```python
from build123d import *

# Parameters (mm, degrees)
SKETCH1_R           = 2.15
BOSS_EXTRUDE1_DEPTH = 4
FILLET1_R           = 2
FILLET3_R           = 1


with BuildPart() as part:
    # Sketch1 → Boss-Extrude1 (new body)
    with BuildSketch(Plane.XY):
        with BuildLine():
            Line((-5e-09, -4), (50.8, -4))
            ThreePointArc((50.8, -4), (53.628427143, -2.828427107), (54.8, 5.1e-08))
            Line((54.8, 5.1e-08), (54.8, 38.1))
            ThreePointArc((54.8, 38.1), (52.588854382, 41.677708764), (48.4, 41.3))
            Line((48.4, 41.3), (25.4, 24.05))
            Line((25.4, 24.05), (2.4, 41.3))
            ThreePointArc((2.4, 41.3), (-1.788854382, 41.677708764), (-4, 38.1))
            Line((-4, 38.1), (-4, 0))
            ThreePointArc((-4, 0), (-2.828427127, -2.828427123), (-5e-09, -4))
        make_face()
        Polygon((46.8, 8), (32.066666667, 19.05), (46.8, 30.1), align=None, mode=Mode.SUBTRACT)
        Circle(SKETCH1_R, mode=Mode.SUBTRACT)
        Polygon((4, 8), (4, 30.1), (18.733333333, 19.05), align=None, mode=Mode.SUBTRACT)
        Polygon((25.4, 14.05), (38.8, 4), (12, 4), align=None, mode=Mode.SUBTRACT)
        with Locations((25.4, 19.05)):
            Circle(SKETCH1_R, mode=Mode.SUBTRACT)
        with Locations((50.8, 0)):
            Circle(SKETCH1_R, mode=Mode.SUBTRACT)
        with Locations((0, 38.1)):
            Circle(SKETCH1_R, mode=Mode.SUBTRACT)
        with Locations((50.8, 38.1)):
            Circle(SKETCH1_R, mode=Mode.SUBTRACT)
    extrude(amount=BOSS_EXTRUDE1_DEPTH)

    # Fillet1
    fillet1_edges = [part.edges().sort_by_distance(p)[0] for p in [
        (18.733333333, 19.05, 2),
        (25.4, 14.05, 2),
        (32.066666667, 19.05, 2),
        (25.4, 24.05, 2),
    ]]
    fillet(fillet1_edges, radius=FILLET1_R)

    # Fillet3
    fillet3_edges = [part.edges().sort_by_distance(p)[0] for p in [
        (4, 30.1, 2),
        (4, 8, 2),
        (12, 4, 2),
        (38.8, 4, 2),
        (46.8, 30.1, 2),
        (46.8, 8, 2),
    ]]
    fillet(fillet3_edges, radius=FILLET3_R)


solid = part.part
```
Geometry: final body of the model. Coordinates: model frame, mm. A direction names the side the tool comes from. Give positions to 0.01 mm unless a question says otherwise; leave off trailing zeros. Order: outer loops, then holes, each group sorted by start corner. A loop starts at its lowest first (then second) coordinate and runs counter-clockwise, first axis right, second up. Notation, with made-up numbers: (75, 64) -> (91, 64) arc R26 cw to (91, 84) -> close; hole circle Ø1 at (18, 46). An arc over 180 degrees is marked (long way). Write each question's results on one line, items separated by ' | '. Start each with the question number.
1) Section C-C (z = 0.7). Count the separate pieces of the cut face and the enclosed holes in it, then the cut area to 3 significant figures.
2) Section D-D (x = 25.4). Return loops of the section in (y, z).
3) First-contact query: pin 1 (1.5 mm diameter, centred on x = 11, y = 30.5, fed in from -Z); pin 2 (2 mm diameter, centred on x = 20.5, z = 1.5, fed in from +Y) (3 decimals); pin 3 (1 mm diameter, centred on x = 21, z = 3, fed in from +Y) (3 decimals); pin 4 (1 mm diameter, centred on x = 36, z = 1, fed in from +Y) (3 decimals). Flat tips, straight axial feed; report the tip coordinate or a pass-through.
4) Line query: line 1 (Y direction, x = 0, z = 1); line 2 (Y direction, x = 25.4, z = 1); line 3 (X direction, y = 27, z = 0.8). Output: solid intervals per line, ascending. Write a range as from..to.
5) Draft query along X for faces 1 (the flat face through (25, -4, 2)), 2 (the flat face through (54.8, 19, 2)), 3 (the cylindrical face through (46.26, 9.11, 2.03)). Return one class per face: pulls with the +X half, pulls with the -X half, needs draft (parallel to the pull), parting line crosses it, or undercut.
6) Section B-B (y = 12). Return loops of the section in (x, z), then the cut area to 3 significant figures.
7) Section A-A (x = 13). Return loops of the section in (y, z).
8) Set-up query: faces 4 (the flat face through (37.653, 33.239, 1.972)), 5 (the cylindrical face through (14, 5, 2)), 6 (the cylindrical face through (-2.859, -2.797, 1.972)). Return all of +Z, -Z, +X, -X, +Y, -Y with unobstructed straight access to the full face (end or side cutting, diameter ignored); none if empty.
Calculated:
1) separate pieces: 1 | enclosed holes: 8 | area: 1,740 mm2
2) outline: (-4, 0) -> (4, 0) -> (4, 4) -> (-4, 4) -> close; (13.55, 0) -> (16.9, 0) -> (16.9, 4) -> (13.55, 4) -> close; (21.2, 0) -> (24.55, 0) -> (24.55, 4) -> (21.2, 4) -> close
3) pin 1: z = 0 | pin 2: y = 28.475 | pin 3: y = 27.725 | pin 4: y = 32.375
4) line 1: -4..-2.15, 2.15..35.95, 40.25..42.1 | line 2: -4..4, 13.55..16.9, 21.2..24.55 | line 3: -4..4, 8.13..21.47, 29.33..42.67, 46.8..54.8
5) face 1: needs draft | face 2: pulls with the +X half | face 3: undercut
6) outline: (-4, 0) -> (4, 0) -> (4, 4) -> (-4, 4) -> close; (9.33, 0) -> (22.67, 0) -> (22.67, 4) -> (9.33, 4) -> close; (28.13, 0) -> (41.47, 0) -> (41.47, 4) -> (28.13, 4) -> close; (46.8, 0) -> (54.8, 0) -> (54.8, 4) -> (46.8, 4) -> close | area: 171 mm2
7) outline: (-4, 0) -> (14.75, 0) -> (14.75, 4) -> (-4, 4) -> close; (23.35, 0) -> (33.35, 0) -> (33.35, 4) -> (23.35, 4) -> close
8) face 4: +Z, -Z, +Y | face 5: +Z, -Z | face 6: +Z, -Z, -X, -Y
